Here's how the part is built. I have some questions about the finished solid (model axes, mm). Coordinates: 2 decimals unless noted, no trailing zeros. Order: outer loops, then holes, each group sorted by start corner. A loop starts at its lowest first (then second) coordinate and runs counter-clockwise, first axis right, second up. Notation, with made-up numbers: (29, 11) - (37, 11) arc R17 cw to (37, 16) - close; hole circle Ø7 at (-27.5, 79). An arc over 180 degrees is marked (long way). Answer as CSV lines item,"result". Start each with the question number.
Q1. Suppose I cut it at D-D (y = -87). Please give me the cut outline in (x, z), then the cut area to 3 significant figures.
Q2. Thinking about a two-plate mould opening in Y: for faces 1 (the face through (72.3, 61.1, 1)), 2 (the face through (116, 83, 0)), which applies, released by +Y, released by -Y, zero draft, split by the parting line, or undercut?
Q3. Suppose I cut it at B-B (z = 0.5). Please give me the cut outline in (x, y).
Q4. For pin 1 Ø4 at (x, y) = (147, 111) entering from -Z, with a flat end and sliding along its axis, tell me the tip position at first contact or that it passes through.
Q5. I need wall thicknesses on line 1 (Y direction, x = 63, z = 0.8); line 2 (X direction, y = -102.5, z = 0.7); line 3 (X direction, y = 59, z = 1.7). Which ranges of each line are inside material? Lowest first, please.
Q6. Suppose I cut it at A-A (y = -36.5). Please give me the cut outline in (x, z).
Q7. Suppose I cut it at C-C (x = 24.5). Please give me the cut outline in (y, z).
from build123d import *

# Parameters (mm, degrees)
SKETCH2_W           = 500
SKETCH2_H           = 500
BOSS_EXTRUDE2_DEPTH = 2
SKETCH5_R           = 50.55
CUT_EXTRUDE1_DEPTH  = 2
SKETCH6_R           = 25
CUT_EXTRUDE2_DEPTH  = 10


with BuildPart() as part:
    # Sketch2 → Boss-Extrude2 (new body)
    with BuildSketch(Plane.XY):
        with Locations((119.822485207, 79.881656805)):
            Rectangle(SKETCH2_W, SKETCH2_H)
    extrude(amount=BOSS_EXTRUDE2_DEPTH)

    # Sketch5 → Cut-Extrude1 (cut)
    with BuildSketch(Plane.XY.offset(2)):
        with Locations((58.842485207, -59.968343195)):
            Circle(SKETCH5_R)
        with Locations((181.142485207, -59.968343195)):
            Circle(SKETCH5_R)
    extrude(amount=-CUT_EXTRUDE1_DEPTH, mode=Mode.SUBTRACT)

    # Sketch6 → Cut-Extrude2 (cut)
    with BuildSketch(Plane.XY.offset(2)):
        with Locations((181.142485207, 40.031656805)):
            Circle(SKETCH6_R)
        with Locations((58.842485207, 40.031656805)):
            Circle(SKETCH6_R)
    extrude(amount=-CUT_EXTRUDE2_DEPTH, mode=Mode.SUBTRACT)


solid = part.part
Here are the results:
1,outline,"(-130.18, 0) - (16.13, 0) - (16.13, 2) - (-130.18, 2) - close; (101.56, 0) - (138.43, 0) - (138.43, 2) - (101.56, 2) - close; (223.86, 0) - (369.82, 0) - (369.82, 2) - (223.86, 2) - close"
1,area,"658 mm²"
2,face 1,"undercut"
2,face 2,"zero draft"
3,outline,"(-130.18, -170.12) - (369.82, -170.12) - (369.82, 329.88) - (-130.18, 329.88) - close; hole circle Ø101.1 at (58.84, -59.97); hole circle Ø50 at (58.84, 40.03); hole circle Ø101.1 at (181.14, -59.97); hole circle Ø50 at (181.14, 40.03)"
4,pin 1,"stops at z = 0"
5,line 1,"y = -170.12 to -110.35, -9.59 to 15.38, 64.68 to 329.88"
5,line 2,"x = -130.18 to 31.52, 86.16 to 153.82, 208.46 to 369.82"
5,line 3,"x = -130.18 to 42.56, 75.13 to 164.86, 197.43 to 369.82"
6,outline,"(-130.18, 0) - (14.07, 0) - (14.07, 2) - (-130.18, 2) - close; (103.61, 0) - (136.37, 0) - (136.37, 2) - (103.61, 2) - close; (225.91, 0) - (369.82, 0) - (369.82, 2) - (225.91, 2) - close"
7,outline,"(-170.12, 0) - (-97.06, 0) - (-97.06, 2) - (-170.12, 2) - close; (-22.88, 0) - (329.88, 0) - (329.88, 2) - (-22.88, 2) - close"
